Source: three-view drawing plus pictorial views. Frame: mm from the lowest corner of the part. A direction names the side the tool comes from. Give positions to 0.01 mm unless a question says otherwise; leave off trailing zeros. Order: outer loops, then holes, each group sorted by start corner. A loop starts at its lowest first (then second) coordinate and runs counter-clockwise, first axis right, second up. Notation, with made-up numbers: M 14.5,40.25 L 30.5,40.25 A18 ccw 30.5,64.25 Z; hole C 18,-11.75 d4. An arc over 180 degrees is marked long. Use CSV: the item, a comma, the result in double quotes. Start each with the question number.
1. Mould query, pull axis Z, two halves, no side actions, for the marked faces 1, 2, 3 and 4. Classes: released by +Z, released by -Z, zero draft, split by the parting line, or undercut.
2. Section query D-D, the plane z = 27. Return the cut outline in (x, y), plus the area to 3 significant figures.
3. Section query C-C, the plane y = 22.5. Return the cut outline in (x, z).
4. Pin query (flat end, axial travel): P1, Ø3, axis at x = 9.5, y = 33, coming from the +Z side; P2, Ø8.5, axis at x = 57.5, y = 70, coming from the +Z side; P3, Ø1, axis at y = 40, z = 31, coming from the +X side; P4, Ø4, axis at x = 15, y = 2.5, coming from the -Z side. Return the tip coordinate at first contact, or that it passes through.
5. Line query: line 1 along Y through (x, z) = (13, 9); line 2 along X through (y, z) = (33.5, 31); line 3 along X through (y, z) = (17, 25). Output: solid intervals per line, ascending. Write a range as [from, to].
6. Section query A-A, the plane z = 44.5. Return the cut outline in (x, y).
7. Section query B-B, the plane x = 17. Return the cut outline in (y, z), plus the area to 3 significant figures.
8. Reachability of the marked faces 5, 6, 7 and 8 from +Z, -Z, +X, -X, +Y, -Y: full face, straight path, thin tool, end or side. Return the list, or none.
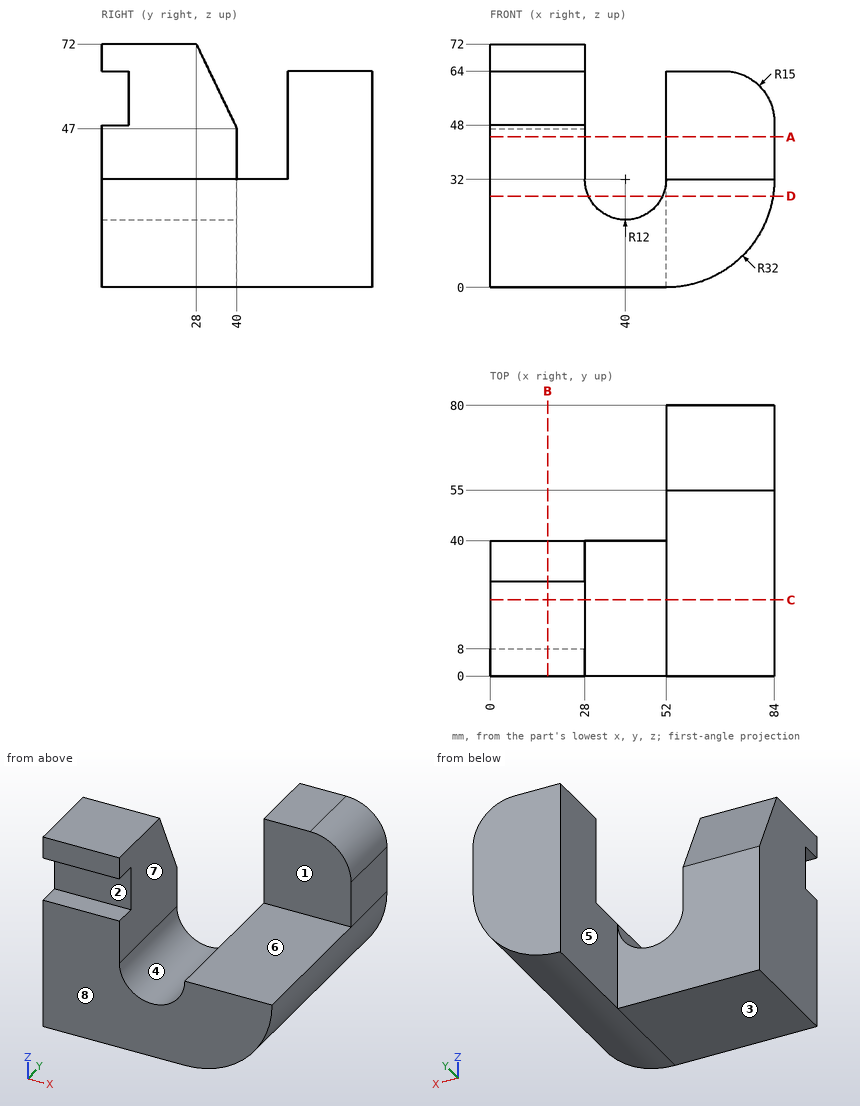
Result set:
1,face 1,"zero draft"
1,face 2,"undercut"
1,face 3,"released by -Z"
1,face 4,"released by +Z"
2,outline,"M 0,0 L 29.09,0 L 29.09,40 L 0,40 Z; M 50.91,0 L 83.61,0 L 83.61,80 L 52,80 L 52,40 L 50.91,40 Z"
2,area,"3,740 mm2"
3,outline,"M 0,0 L 52,0 A32 ccw 84,32 L 52,32 A12 cw 28,32 L 28,72 L 0,72 Z"
4,P1,"z = 64.71"
4,P2,"z = 64"
4,P3,"x = 84"
4,P4,"z = 0"
5,line 1,"[0, 40]"
5,line 2,"[0, 28.04], [51.96, 83.98]"
5,line 3,"[0, 30.25], [49.75, 83.22]"
6,outline,"M 0,0 L 28,0 L 28,40 L 0,40 Z; M 52,55 L 84,55 L 84,80 L 52,80 Z"
7,outline,"M 0,0 L 40,0 L 40,47 L 28,72 L 0,72 L 0,64 L 8,64 L 8,48 L 0,48 Z"
7,area,"2,600 mm2"
8,face 5,"+Z, -Z, -X, +Y"
8,face 6,"+Z, +X, -Y"
8,face 7,"+Z, +X, +Y, -Y"
8,face 8,"+Z, -Z, +X, -X, -Y"
